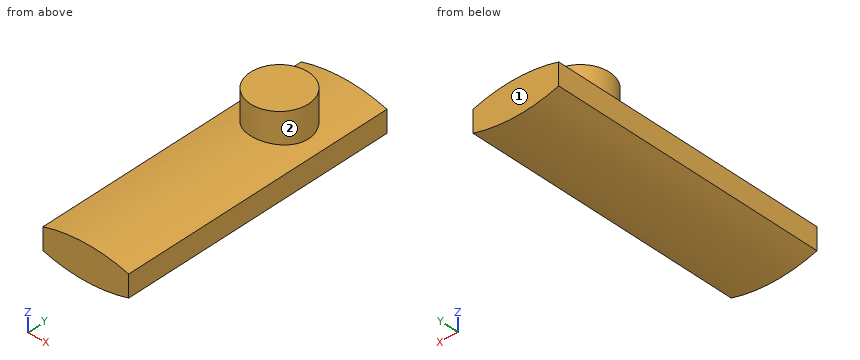
from build123d import *

# Parameters (mm, degrees)
F1_DEPTH = 76.2
F2_R     = 15.891497
F3_DEPTH = 25.4


with BuildPart() as f1:
    # F0 (on Front) → F1 (new body, symmetric)
    with BuildSketch(Plane.XZ):
        with BuildLine():
            ThreePointArc((23.529917, 6.007624), (0, 9.508228), (-23.529917, 6.007624))
            Line((-23.529917, 6.007624), (-23.529917, -6.007624))
            ThreePointArc((-23.529917, -6.007624), (0, -9.508228), (23.529917, -6.007624))
            Line((23.529917, -6.007624), (23.529917, 6.007624))
        make_face()
    extrude(amount=F1_DEPTH, both=True)

    # F2 (on Top) → F3 (join)
    with BuildSketch(Plane.XY):
        with Locations((0, 38.051773)):
            Circle(F2_R)
    extrude(amount=F3_DEPTH)


solid = f1.part
Verification items for the finished model (mm, model axes). Face numbers are marked on the shaded views. A direction names the side the tool comes from. Coordinates: 2 decimals unless noted, no trailing zeros. Write each loop counter-clockwise with the first axis right and the second up, starting at its lowest first coordinate (ties: lowest second). Pieces come first, ordered by that corner, then holes. Notation, with made-up numbers: M 55,72.25 L 73,72.25 A21 cw 73,80.25 Z; hole C 80,52 d4. An arc over 180 degrees is marked long. Use a Markdown table: item, result.
Q1. Sectioned sample at B-B, the plane y = -42. Record the boundary of the cut face in (x, z).
Reply:
| item | result |
|---|---|
| outline | M -23.53,-6.01 A80.83 ccw 23.53,-6.01 L 23.53,6.01 A80.83 ccw -23.53,6.01 Z |
Q2. Sectioned sample at D-D, the plane x = 10. Record the boundary of the cut face in (y, z), plus the area to 3 significant figures.
Reply:
| item | result |
|---|---|
| outline | M -76.2,-8.89 L 76.2,-8.89 L 76.2,8.89 L 50.4,8.89 L 50.4,25.4 L 25.7,25.4 L 25.7,8.89 L -76.2,8.89 Z |
| area | 3,120 mm² |
Q3. Thickness scan on line 1 (Y direction, x = 0.5, z = 18.5); line 2 (Z direction, x = 0.5, y = 15.5); line 3 (Z direction, x = 5, y = 14.5). Record the ranges inside material, lowest first.
Reply:
| item | result |
|---|---|
| line 1 | y = 22.17 to 53.94 |
| line 2 | z = -9.51 to 9.51 |
| line 3 | z = -9.35 to 9.35 |
Q4. Sectioned sample at A-A, the plane x = 0. Record the boundary of the cut face in (y, z), plus the area to 3 significant figures.
Reply:
| item | result |
|---|---|
| outline | M -76.2,-9.51 L 76.2,-9.51 L 76.2,9.51 L 53.94,9.51 L 53.94,25.4 L 22.16,25.4 L 22.16,9.51 L -76.2,9.51 Z |
| area | 3,400 mm² |
Q5. Set-up check for the marked faces 1 and 2: record each of +Z, -Z, +X, -X, +Y, -Y from which the full face is reachable in a straight line by a thin tool's end or side.
Reply:
| item | result |
|---|---|
| face 1 | +Z, -Z, +X, -X, +Y |
| face 2 | +Z |
Q6. Go/stop test with flat-tipped pins: P1, Ø12, axis at x = -7, y = 2, coming from the -Z side; P2, Ø5, axis at x = -8, y = -39.5, coming from the -Z side; P3, Ø10, axis at x = 3, z = 10, coming from the +Y side; P4, Ø3, axis at x = -10.5, y = 37.5, coming from the -Z side. Record where each tip stops, or that it passes through.
Reply:
| item | result |
|---|---|
| P1 | stops at z = -9.5 |
| P2 | stops at z = -9.32 |
| P3 | stops at y = 76.2 |
| P4 | stops at z = -9.01 |
Q7. Sectioned sample at C-C, the plane z = 18. Record the boundary of the cut face in (x, y).
Reply:
| item | result |
|---|---|
| outline | C 0,38.05 d31.78 |
